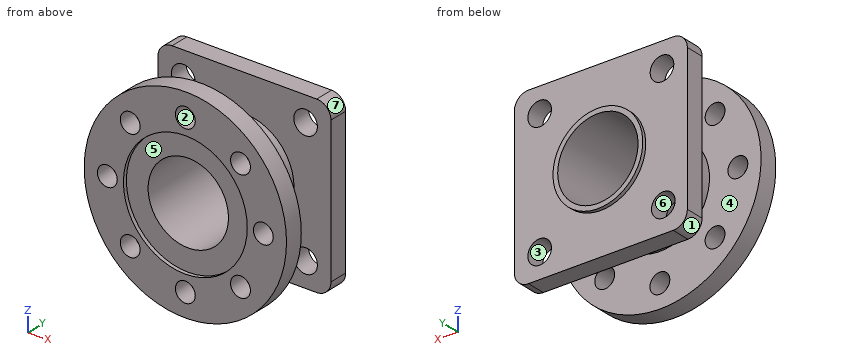
from build123d import *

# Parameters (mm, degrees)
F0_W      = 183
F0_H      = 183
F0_R      = 42.5
F1_DEPTH  = 20
F2_R      = 15
F3_D      = 25
F3_DEPTH  = 31
F3_TIP    = 7.5107577378
F4_R      = 47.5
F4_R_2    = 42.5
F5_DEPTH  = 4
F6_R      = 52.5
F6_R_2    = 42.5
F7_DEPTH  = 60
F8_R      = 107
F8_R_2    = 42.5
F9_DEPTH  = 20
F10_D     = 21
F10_DEPTH = 20
F10_TIP   = 6.3090364998
F11_R     = 65.5
F12_DEPTH = 4


with BuildPart() as f1:
    # F0 (on Front) → F1 (new body)
    with BuildSketch(Plane.XZ):
        Rectangle(F0_W, F0_H)
        Circle(F0_R, mode=Mode.SUBTRACT)
    extrude(amount=F1_DEPTH)

    # F2
    f2_edges = [f1.edges().sort_by_distance(p)[0] for p in [
        (-91.5, -10, 91.5),
        (91.5, -10, 91.5),
        (91.5, -10, -91.5),
        (-91.5, -10, -91.5),
    ]]
    fillet(f2_edges, radius=F2_R)

    # F3
    with Locations(Plane(origin=(0, 0, 0), x_dir=(1, 0, 0), z_dir=(0, 1, 0))):
        with Locations((64.7000986303, 65.4056361274), (64.6997307877, -65.406), (-64.7000986303, -65.4056361274), (-66.1115414671, 63.9941972606)):
            Hole(F3_D / 2, depth=F3_DEPTH)
            with Locations((0, 0, -(F3_DEPTH + F3_TIP / 2))):  # 118° drill point
                Cone(0, F3_D / 2, F3_TIP, mode=Mode.SUBTRACT)

    # F4 (on face) → F5 (join)
    with BuildSketch(Plane.XZ):
        Circle(F4_R)
        Circle(F4_R_2, mode=Mode.SUBTRACT)
    extrude(amount=-F5_DEPTH)

    # F6 (on face) → F7 (join)
    with BuildSketch(Plane.XZ.offset(20)):
        Circle(F6_R)
        Circle(F6_R_2, mode=Mode.SUBTRACT)
    extrude(amount=F7_DEPTH)

    # F8 (on face) → F9 (join)
    with BuildSketch(Plane.XZ.offset(80)):
        Circle(F8_R)
        Circle(F8_R_2, mode=Mode.SUBTRACT)
    extrude(amount=F9_DEPTH)

    # F10 (one way)
    with BuildSketch(Plane(origin=(0, -80, 0), x_dir=(1, 0, 0), z_dir=(0, 1, 0))):
        with Locations((82.5, 0), (58.3363094479, -58.3363094479), (0, -82.5), (-58.3363094479, -58.3363094479), (-82.5, 0), (-58.3363094479, 58.3363094479), (0, 82.5), (58.3363094479, 58.3363094479)):
            Circle(F10_D / 2)
    extrude(amount=-F10_DEPTH, mode=Mode.SUBTRACT)
    with Locations(Plane(origin=(0, -80, 0), x_dir=(1, 0, 0), z_dir=(0, 1, 0))):
        with Locations((82.5, 0), (58.3363094479, -58.3363094479), (0, -82.5), (-58.3363094479, -58.3363094479), (-82.5, 0), (-58.3363094479, 58.3363094479), (0, 82.5), (58.3363094479, 58.3363094479)):
            with Locations((0, 0, -(F10_DEPTH + F10_TIP / 2))):  # 118° drill point
                Cone(0, F10_D / 2, F10_TIP, mode=Mode.SUBTRACT)

    # F11 (on face) → F12 (cut)
    with BuildSketch(Plane.XZ.offset(100)):
        Circle(F11_R)
    extrude(amount=-F12_DEPTH, mode=Mode.SUBTRACT)


solid = f1.part
Design review of the part built by this model. Coordinates are the model's own, in mm. Face numbers are marked on the shaded views. A direction names the side the tool comes from. Coordinates: 2 decimals unless noted, no trailing zeros. Loops run counter-clockwise (first coordinate to the right, second up) from the corner with the lowest first, then second, coordinate; pieces in that order, holes last. Notation, with made-up numbers: M 34,-21.5 L 40,-21.5 A22 ccw 40,-10.5 Z; hole C -40,87.5 d9. An arc over 180 degrees is marked long. Answer as CSV lines item,"result".
Item 1: Add section A-A on z = 0. Count the separate pieces of the cut face and the enclosed holes in it, plus the area to 3 significant figures.
Answer list:
separate pieces,"4"
enclosed holes,"0"
area,"4,760 mm²"
Item 2: The part is to be moulded in two halves that separate along X. For the marked faces 1, 2, 3 and 4, say which applies: pulls with the +X half, pulls with the -X half, needs draft (parallel to the pull), parting line crosses it, or undercut.
Answer list:
face 1,"pulls with the -X half"
face 2,"undercut"
face 3,"undercut"
face 4,"needs draft"
Item 3: For P1, Ø22, axis at y = -8, z = 14, coming from the +X side; P2, Ø6, axis at x = 6, y = -6, coming from the -Z side; P3, Ø6, axis at y = -6.5, z = 38, coming from the -X side; P4, Ø4, axis at y = -23.5, z = -56.5, coming from the -X side, all flat-tipped, find the tip position at first contact; note any pin that passes through.
Answer list:
P1,"x = 91.5"
P2,"z = -91.5"
P3,"x = -91.5"
P4,"through"
Item 4: Add section C-C on x = -82.5. State the section outline as (y, z) points.
Answer list:
outline,"M -100,-68.14 L -80,-68.14 L -80,-10.5 L -100,-10.5 Z; M -100,10.5 L -80,10.5 L -80,68.14 L -100,68.14 Z; M -20,-90.25 L 0,-90.25 L 0,90.25 L -20,90.25 Z"
Item 5: Add section D-D on y = -11.5. State the section outline as (x, z) points.
Answer list:
outline,"M -91.5,-76.5 A15 ccw -76.5,-91.5 L 76.5,-91.5 A15 ccw 91.5,-76.5 L 91.5,76.5 A15 ccw 76.5,91.5 L -76.5,91.5 A15 ccw -91.5,76.5 Z; hole C -66.11,-63.99 d25; hole C -64.7,65.41 d25; hole C 0,0 d85; hole C 64.7,-65.41 d25; hole C 64.7,65.41 d25"
Item 6: For probe 1 along Y at (x, z) = (-21.5, -68.5); probe 2 along X at (y, z) = (-10, 67); probe 3 along X at (y, z) = (-78, 6), list the stretches that pass through material, from the lowest coordinate up.
Answer list:
probe 1,"-100 to -80, -20 to 0"
probe 2,"-91.5 to -77.1, -52.3 to 52.3, 77.1 to 91.5"
probe 3,"-52.16 to -42.07, 42.07 to 52.16"
Item 7: Machinability: for the marked faces 5, 6 and 7, which of the approach directions +Z, -Z, +X, -X, +Y, -Y give a long, thin tool a straight path to every point of the face, cutting with its end or side? Answer none if there is none.
Answer list:
face 5,"-Y"
face 6,"+Y"
face 7,"+Z, +X, +Y, -Y"
